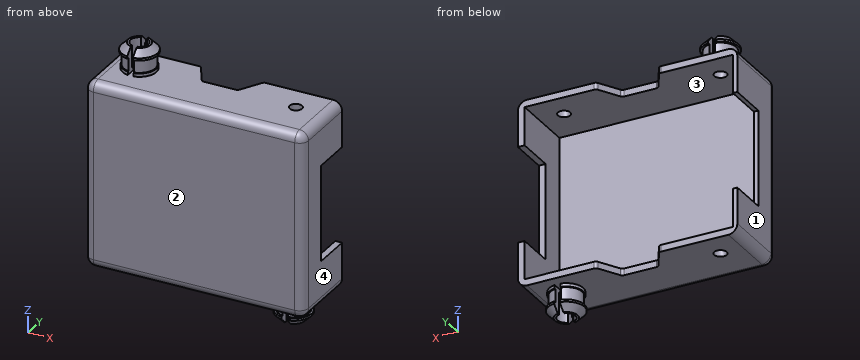
from build123d import *

# Parameters (mm, degrees)
SKETCH1_W                                    = 97.5
SKETCH1_H                                    = 82.5
BOSS_EXTRUDE1_DEPTH                          = 32
SHELL1_T                                     = -3
FILLET1_R                                    = 4
CUT_EXTRUDE1_START                           = -1
SKETCH4_W                                    = 76.5
SKETCH4_H                                    = 29
CUT_EXTRUDE1_DEPTH                           = 83.5
CUT_EXTRUDE2_REACH                           = 133.668
SKETCH5_W                                    = 42.5
SKETCH5_H                                    = 17.5
CUT_EXTRUDE3_REACH                           = 133.668
FILLET2_R                                    = 1.5
CUT_EXTRUDE4_START                           = -82.5
SKETCH7_R                                    = 2.75
CUT_EXTRUDE4_DEPTH                           = 82.5
SKETCH9_R                                    = 7.5
SKETCH9_R_2                                  = 2.75
BOSS_EXTRUDE3_DEPTH                          = 1.5
CUT_EXTRUDE5_REACH                           = 133.668
SKETCH11_W                                   = 2.5
SKETCH11_H                                   = 16
MIRROR2_AT_THE_SECOND_PLANE_COPY_1_SKETC_R   = 7.5
MIRROR2_AT_THE_SECOND_PLANE_COPY_1_SKETC_R_2 = 2.75
MIRROR2_AT_THE_SECOND_PLANE_COPY_1_DEPTH     = 1.5
MIRROR2_AT_THE_SECOND_PLANE_COPY_3_REACH     = 133.668
MIRROR2_AT_THE_SECOND_PLANE_COPY_3_SKETC_W   = 2.5
MIRROR2_AT_THE_SECOND_PLANE_COPY_3_SKETC_H   = 16
SKETCH12_W                                   = 25.238507428
SKETCH12_H                                   = 22.458767107
CUT_EXTRUDE6_DEPTH                           = 11.5
CUT_EXTRUDE7_REACH                           = 141.163
SKETCH13_W                                   = 31.509123874
SKETCH13_H                                   = 19.339493898


with BuildPart() as part:
    # Sketch1 → Boss-Extrude1 (new body)
    with BuildSketch(Plane(origin=(0, 0, 0), x_dir=(1, 0, 0), z_dir=(0, 1, 0))):
        with Locations((48.75, 41.25)):
            Rectangle(SKETCH1_W, SKETCH1_H)
    extrude(amount=BOSS_EXTRUDE1_DEPTH)

    # Shell1
    shell1_openings = [part.faces().sort_by_distance(p)[0] for p in [
        (48.75, 32, -41.25),
    ]]
    offset(amount=SHELL1_T, openings=shell1_openings, kind=Kind.INTERSECTION)

    # Fillet1
    fillet1_edges = [part.edges().sort_by_distance(p)[0] for p in [
        (48.75, 0, -82.5),
        (97.5, 0, -41.25),
        (48.75, 0, 0),
        (0, 0, -41.25),
        (0, 16, -82.5),
        (97.5, 16, -82.5),
        (97.5, 16, 0),
        (0, 16, 0),
    ]]
    fillet(fillet1_edges, radius=FILLET1_R)

    # Sketch4 → Cut-Extrude1 (cut)
    with BuildSketch(Plane(origin=(3, 0, 0), x_dir=(0, 0, -1), z_dir=(1, 0, 0)).offset(CUT_EXTRUDE1_START)):
        with Locations((41.25, 17.5)):
            Rectangle(SKETCH4_W, SKETCH4_H)
    extrude(amount=CUT_EXTRUDE1_DEPTH, mode=Mode.SUBTRACT)

    # Cut-Extrude2: up to this face of the body (flat: up to its plane)
    cut_extrude2_end = Plane(part.part.faces().sort_by_distance((0, 18, -41.25))[0])
    # Sketch5 → Cut-Extrude2 (cut, up to the picked face)
    with BuildSketch(Plane(origin=(97.5, 0, 0), x_dir=(0, 0, -1), z_dir=(1, 0, 0)), mode=Mode.PRIVATE) as cut_extrude2_sk1:
        with Locations((41.25, 23.25)):
            Rectangle(SKETCH5_W, SKETCH5_H)
    cut_extrude2_tool1 = split(extrude(cut_extrude2_sk1.sketch, amount=-CUT_EXTRUDE2_REACH, mode=Mode.PRIVATE), bisect_by=cut_extrude2_end, keep=Keep.BOTH, mode=Mode.PRIVATE)
    add(cut_extrude2_tool1.solids().sort_by(Axis((97.5, 23.25, -41.25), (-1, 0, 0)))[0], mode=Mode.SUBTRACT)

    # Cut-Extrude3: up to this face of the body (flat: up to its plane)
    cut_extrude3_end = Plane(part.part.faces().sort_by_distance((48.75, 18, -82.5))[0])
    # Sketch6 → Cut-Extrude3 (cut, up to the picked face)
    with BuildSketch(Plane.XY, mode=Mode.PRIVATE) as cut_extrude3_sk1:
        Polygon((40.75, 21.5), (56.75, 21.5), (62.75, 32), (34.75, 32), align=None)
    cut_extrude3_tool1 = split(extrude(cut_extrude3_sk1.sketch, amount=-CUT_EXTRUDE3_REACH, mode=Mode.PRIVATE), bisect_by=cut_extrude3_end, keep=Keep.BOTH, mode=Mode.PRIVATE)
    add(cut_extrude3_tool1.solids().sort_by(Axis((48.75, 27.227273, 0), (0, 0, -1)))[0], mode=Mode.SUBTRACT)

    # Fillet2
    fillet2_edges = [part.edges().sort_by_distance(p)[0] for p in [
        (40.75, 21.5, -1.5),
        (34.75, 32, -1.5),
        (62.75, 32, -1.5),
        (56.75, 21.5, -1.5),
        (40.75, 21.5, -81),
        (34.75, 32, -81),
        (62.75, 32, -81),
        (56.75, 21.5, -81),
    ]]
    fillet(fillet2_edges, radius=FILLET2_R)

    # Sketch7 → Cut-Extrude4 (cut)
    with BuildSketch(Plane.XY.offset(CUT_EXTRUDE4_START)):
        with Locations((14, 19.75)):
            Circle(SKETCH7_R)
        with Locations((83.5, 19.75)):
            Circle(SKETCH7_R)
    extrude(amount=CUT_EXTRUDE4_DEPTH, mode=Mode.SUBTRACT)

    # Sketch9 → Boss-Extrude3 (add)
    with BuildSketch(Plane.XY):
        with Locations(Location((14, 19.75, 0), (0, 0, 180))):
            Circle(SKETCH9_R)
        with Locations((14, 19.75)):
            Circle(SKETCH9_R_2, mode=Mode.SUBTRACT)
    boss_extrude3 = extrude(amount=BOSS_EXTRUDE3_DEPTH)

    # Sketch10 → Revolve1 (revolve)
    with BuildSketch(Plane.ZY.offset(-14), mode=Mode.PRIVATE) as revolve1_sk:
        Polygon((11.5, 24.75), (8.5, 27.75), (7.5, 27.75), (7.5, 26.75), (1.5, 26.75), (1.5, 23.75), (11.5, 23.75), align=None)
    revolve1 = revolve(revolve1_sk.sketch.rotate(Axis((14, 19.75, 0), (0, 0, 1)), 90), axis=Axis((14, 19.75, 0), (0, 0, 1)))

    # Cut-Extrude5: up to this face of the body (flat: up to its plane)
    cut_extrude5_end = Plane(part.part.faces().sort_by_distance((18.141421356, 19.75, 11.5))[0])
    # Sketch11 → Cut-Extrude5 (cut, up to the picked face)
    with BuildSketch(Plane.XY, mode=Mode.PRIVATE) as cut_extrude5_sk1:
        with Locations((14, 19.75)):
            Rectangle(SKETCH11_W, SKETCH11_H)
    cut_extrude5_tool1 = split(extrude(cut_extrude5_sk1.sketch, amount=CUT_EXTRUDE5_REACH, mode=Mode.PRIVATE), bisect_by=cut_extrude5_end, keep=Keep.BOTH, mode=Mode.PRIVATE)
    cut_extrude5 = cut_extrude5_tool1.solids().sort_by(Axis((14, 19.75, 0), (0, 0, 1)))[0]
    add(cut_extrude5, mode=Mode.SUBTRACT)

    # Mirror2: Boss-Extrude3, Revolve1, Cut-Extrude5 across plane
    add(boss_extrude3.mirror(Plane.ZY.offset(-48.25)))
    add(revolve1.mirror(Plane.ZY.offset(-48.25)))
    add(cut_extrude5.mirror(Plane.ZY.offset(-48.25)), mode=Mode.SUBTRACT)

    # Mirror2 at the second plane: Boss-Extrude3, Revolve1, Cut-Extrude5 across plane
    add(boss_extrude3.mirror(Plane.XY.offset(-41.25)))
    add(revolve1.mirror(Plane.XY.offset(-41.25)))
    add(cut_extrude5.mirror(Plane.XY.offset(-41.25)), mode=Mode.SUBTRACT)

    # Mirror2 at the second plane copy 1 sketc → Mirror2 at the second plane copy 1 (add)
    with BuildSketch(Plane(origin=(96.5, 0, -82.5), x_dir=(-1, 0, 0), z_dir=(0, 0, -1))):
        with Locations(Location((14, 19.75, 0), (0, 0, 180))):
            Circle(MIRROR2_AT_THE_SECOND_PLANE_COPY_1_SKETC_R)
        with Locations((14, 19.75)):
            Circle(MIRROR2_AT_THE_SECOND_PLANE_COPY_1_SKETC_R_2, mode=Mode.SUBTRACT)
    extrude(amount=MIRROR2_AT_THE_SECOND_PLANE_COPY_1_DEPTH)

    # Mirror2 at the second plane copy 2 sketc → Mirror2 at the second plane copy 2 (revolve)
    with BuildSketch(Plane(origin=(82.5, 0, -82.5), x_dir=(0, 0, -1), z_dir=(1, 0, 0))):
        Polygon((11.5, 24.75), (8.5, 27.75), (7.5, 27.75), (7.5, 26.75), (1.5, 26.75), (1.5, 23.75), (11.5, 23.75), align=None)
    revolve(axis=Axis((82.5, 19.75, -82.5), (0, 0, -1)))

    # Mirror2 at the second plane copy 3: up to this face of the body (flat: up to its plane)
    mirror2_at_the_second_plane_copy_3_end = Plane(part.part.faces().sort_by_distance((78.358578644, 19.75, -94))[0])
    # Mirror2 at the second plane copy 3 sketc → Mirror2 at the second plane copy 3 (cut, up to the picked face)
    with BuildSketch(Plane(origin=(96.5, 0, -82.5), x_dir=(-1, 0, 0), z_dir=(0, 0, -1)), mode=Mode.PRIVATE) as mirror2_at_the_second_plane_copy_3_sk1:
        with Locations((14, 19.75)):
            Rectangle(MIRROR2_AT_THE_SECOND_PLANE_COPY_3_SKETC_W, MIRROR2_AT_THE_SECOND_PLANE_COPY_3_SKETC_H)
    mirror2_at_the_second_plane_copy_3_tool1 = split(extrude(mirror2_at_the_second_plane_copy_3_sk1.sketch, amount=MIRROR2_AT_THE_SECOND_PLANE_COPY_3_REACH, mode=Mode.PRIVATE), bisect_by=mirror2_at_the_second_plane_copy_3_end, keep=Keep.BOTH, mode=Mode.PRIVATE)
    add(mirror2_at_the_second_plane_copy_3_tool1.solids().sort_by(Axis((82.5, 19.75, -82.5), (0, 0, -1)))[0], mode=Mode.SUBTRACT)

    # Sketch12 → Cut-Extrude6 (cut)
    with BuildSketch(Plane(origin=(0, 0, -82.5), x_dir=(-1, 0, 0), z_dir=(0, 0, -1))):
        with Locations((-16.619253714, 19.183530238)):
            Rectangle(SKETCH12_W, SKETCH12_H)
    extrude(amount=CUT_EXTRUDE6_DEPTH, mode=Mode.SUBTRACT)

    # Sketch13 → Cut-Extrude7 (cut, up to next)
    with BuildSketch(Plane.XY, mode=Mode.PRIVATE) as cut_extrude7_sk1:
        with Locations((77.745438063, 20.1193122)):
            Rectangle(SKETCH13_W, SKETCH13_H)
    cut_extrude7_tool1 = extrude(cut_extrude7_sk1.sketch, amount=CUT_EXTRUDE7_REACH, mode=Mode.PRIVATE) & part.part
    add(cut_extrude7_tool1.solids().sort_by_distance((77.745438, 20.119312, 0))[0], mode=Mode.SUBTRACT)
    add(cut_extrude7_tool1.solids().sort_by_distance((77.745438, 20.119312, 0))[1], mode=Mode.SUBTRACT)


solid = part.part
Here's how the part is built. I have some questions about the finished solid (model axes, mm). Face numbers are marked on the shaded views. Coordinates: 2 decimals unless noted, no trailing zeros. Order: outer loops, then holes, each group sorted by start corner. A loop starts at its lowest first (then second) coordinate and runs counter-clockwise, first axis right, second up. Notation, with made-up numbers: (-35, 57.5) -> (-11, 57.5) arc R19 cw to (-11, 78.5) -> close; hole circle Ø7 at (39, 44.5). An arc over 180 degrees is marked (long way). Answer in a Markdown table with one row per item.
(1) I want a section at C-C on x = 27. List the corners of the cut face in (y, z) for me, then the cut area to 3 significant figures.
Answer key:
| item | result |
|---|---|
| outline | (0, -78.5) arc R4 ccw to (4, -82.5) -> (32, -82.5) -> (32, -79.5) -> (3, -79.5) -> (3, -3) -> (32, -3) -> (32, 0) -> (4, 0) arc R4 ccw to (0, -4) -> close |
| area | 415 mm^2 |
(2) Will these pins go through, and if not, where does the flat tip stop? pin 1 Ø8 at (x, y) = (44, 13.5) entering from -Z; pin 2 Ø2.5 at (y, z) = (25.5, 6.5) entering from -X (3 decimals); pin 3 Ø1 at (x, z) = (29, -81) entering from -Y; pin 4 Ø8 at (y, z) = (7, -69.5) entering from -X.
Answer key:
| item | result |
|---|---|
| pin 1 | z = -82.5 |
| pin 2 | x = 7.755 |
| pin 3 | y = 0.54 |
| pin 4 | x = 0 |
(3) I want a section at B-B on z = -65.5. List the corners of the cut face in (x, y) for me, then the cut area to 3 significant figures.
Answer key:
| item | result |
|---|---|
| outline | (0, 4) arc R4 ccw to (4, 0) -> (93.5, 0) arc R4 ccw to (97.5, 4) -> (97.5, 32) -> (94.5, 32) -> (94.5, 3) -> (2, 3) -> (2, 32) -> (0, 32) -> close |
| area | 431 mm^2 |
(4) Please list where these lines run through material, in increasing order: probe 1 along Z at (x, y) = (92, 26.5); probe 2 along X at (y, z) = (23, -69); probe 3 along X at (y, z) = (19.75, -81.15).
Answer key:
| item | result |
|---|---|
| probe 1 | -82.5 to -79.5, -3 to 0 |
| probe 2 | 0 to 2, 94.5 to 97.5 |
| probe 3 | 1 to 11.25, 16.75 to 80.75, 86.25 to 96.5 |
(5) I want a section at A-A on x = 14. List the corners of the cut face in (y, z) for me.
Answer key:
| item | result |
|---|---|
| outline | (0, -78.5) arc R4 ccw to (4, -82.5) -> (17, -82.5) -> (17, -79.5) -> (3, -79.5) -> (3, -3) -> (17, -3) -> (17, 0) -> (4, 0) arc R4 ccw to (0, -4) -> close; (22.5, -82.5) -> (32, -82.5) -> (32, -79.5) -> (22.5, -79.5) -> close; (22.5, -3) -> (32, -3) -> (32, 0) -> (22.5, 0) -> close |
(6) Thinking about a two-plate mould opening in X: for the marked faces 1, 2, 3 and 4, which applies, +X half, -X half, draft (parallel to the pull), parting line (faces both ways), or undercut?
Answer key:
| item | result |
|---|---|
| face 1 | -X half |
| face 2 | draft |
| face 3 | undercut |
| face 4 | +X half |
(7) I want a section at D-D on y = 19.75. Count the separate pieces of the cut face and the enclosed holes in it, then the cut area to 3 significant figures.
Answer key:
| item | result |
|---|---|
| separate pieces | 6 |
| enclosed holes | 0 |
| area | 822 mm^2 |
